Can you work these out from the model? Positions are in its coordinate system, mm. A direction names the side the tool comes from. Round coordinates to 2 decimals unless told otherwise and drop trailing zeros. Order: outer loops, then holes, each group sorted by start corner. A loop starts at its lowest first (then second) coordinate and runs counter-clockwise, first axis right, second up. Notation, with made-up numbers: M -33.75,20 L -20.75,20 A6 cw -20.75,27 Z; hole C -12,60 d1. An arc over 180 degrees is marked long. One line per question, with ' | ' between items.
Autodesk Inventor part; units mm, degrees
ref_plane "YZ Plane" through (0, 0, 0) normal (1, 0, 0) x (0, 1, 0)
ref_plane "XZ Plane" through (0, 0, 0) normal (0, 1, 0) x (-1, 0, 0)
ref_plane "XY Plane" through (0, 0, 0) normal (0, 0, 1) x (1, 0, 0)
sketch "Sketch1" plane through (0, 0, 0) normal (0, 0, 1) x (1, 0, 0)
  line L0 (0, 0) -> (0, -43.18)
  line L1 (0, 0) -> (12.2773, 16)
  line L2 (0, 0) -> (20.1676, 0) construction
  circle A0 centre (12.2773, 16) radius 1.651
  circle A1 centre (0, 0) radius 1.651
  line L3 (10.0328, 17.2474) -> (-2.54, 0.8622)
  line L4 (-2.54, 0.8622) -> (-2.54, -43.18)
  line L5 (14.063, 14.1549) -> (2.54, -0.8622)
  line L6 (2.54, -0.8622) -> (2.54, -43.18)
  line L7 (10.0328, 17.2474) -> (11.9656, 19.7663)
  line L8 (11.9656, 19.7663) -> (15.9959, 16.6738)
  line L9 (15.9959, 16.6738) -> (14.063, 14.1549)
  line L10 (-2.54, -43.18) -> (2.54, -43.18)
  dimension "d0" = 43.18
  dimension "d1" = 20.1676
  dimension "d2" = 52.5
  dimension "d3" = 3.302
  dimension "d4" = 3.302
  dimension "d5" = 2.54
  dimension "d6" = 2.54
  dimension "d7" = 3.175
extrude "Extrusion1" add sketch "Sketch1" along normal blind 5.9182
fillet "Fillet1" radius 3.175 6 edges at (11.9656, 19.7663, 2.9591) (15.9959, 16.6738, 2.9591) (-2.54, 0.8622, 2.9591) (2.54, -0.8622, 2.9591) (2.54, -43.18, 2.9591) (-2.54, -43.18, 2.9591)
sketch "Sketch2" plane through (0, 0, 0) normal (0, 0, -1) x (-1, 0, 0)
  line L0 (-2.54, -40.005) -> (-2.54, -1.94)
  line L1 (-2.54, -11.43) -> (2.54, -11.43)
  line L2 (2.54, -0.2156) -> (2.54, -40.2701)
  arc A0 (-2.54, -40.005) -> (0.635, -43.18) centre (0.635, -40.005) ccw
  circle A1 centre (0, 0) radius 1.651
  circle A2 centre (-12.2773, 16) radius 1.651
  arc A3 (0.635, -43.18) -> (2.54, -40.2701) centre (-0.635, -40.2701) ccw
  line L3 (2.54, -0.2156) -> (2.54, -40.2701)
  arc A4 (2.54, -0.2156) -> (1.8839, 1.7173) centre (-0.635, -0.2156) ccw
  line L4 (-10.0328, 17.2474) -> (1.8839, 1.7173)
  arc A5 (-10.0328, 17.2474) -> (-14.4845, 17.8335) centre (-12.5517, 15.3146) ccw
  arc A6 (-14.4845, 17.8335) -> (-14.2244, 14.3652) centre (-11.7055, 16.298) ccw
  line L5 (-3.1961, -0.0072) -> (-14.2244, 14.3652)
  arc A7 (-2.54, -1.94) -> (-3.1961, -0.0072) centre (-5.715, -1.94) ccw
  line L6 (-2.54, -40.005) -> (-2.54, -1.94)
  arc A8 (-2.54, -40.005) -> (0.635, -43.18) centre (0.635, -40.005) ccw
  point P0 (0.635, -43.18)
  dimension "d11" = 31.75
extrude "Extrusion2" add sketch "Sketch2" along normal blind 8.255 contours L0 L1 L2 A3 A0
fillet "Fillet2" radius 3.175 2 edges at (0, -11.43, 0) (0, -11.43, -8.255)
sketch "Sketch3" plane through (2.54, -40.005, 5.9182) normal (1, 0, 0) x (0, 0, -1)
  circle A0 centre (5.9182, 1.6434) radius 2
  circle A1 centre (5.9182, 25.1399) radius 2
  arc A2 (14.1732, 25.4) -> (10.9982, 28.575) centre (10.9982, 25.4) ccw
  line L0 (9.0932, 28.575) -> (10.9982, 28.575)
  arc A3 (5.9182, 31.75) -> (9.0932, 28.575) centre (9.0932, 31.75) ccw
  line L1 (5.9182, 31.75) -> (5.9182, 38.065)
  line L2 (0, 38.065) -> (5.9182, 38.065)
  line L3 (0, 0) -> (0, 38.065)
  line L4 (0, 0) -> (14.1732, 0)
  line L5 (14.1732, 25.4) -> (14.1732, 0)
  circle A4 centre (10.9982, 12.7) radius 2
  line L6 (5.9182, 1.6434) -> (10.9982, 12.7)
  line L7 (10.9982, 12.7) -> (5.9182, 25.1399)
  line L8 (4.9924, 24.7618) -> (9.9085, 12.7234)
  line L9 (9.9085, 12.7234) -> (5.0095, 2.0609)
  line L10 (6.844, 25.518) -> (12.0879, 12.6766)
  line L11 (12.0879, 12.6766) -> (6.8269, 1.2259)
  point P0 (5.9182, 40.005)
  point P1 (5.6472, 23.1583)
  point P2 (9.4176, 13.9254)
  point P3 (9.3664, 11.5436)
  point P4 (5.7326, 3.6348)
  point P5 (7.55, 2.7998)
  point P6 (11.1838, 10.7086)
  point P7 (11.2692, 14.6816)
  point P8 (7.4988, 23.9144)
  dimension "d15" = 4
  dimension "d16" = 4
  dimension "d17" = 4
  dimension "d18" = 1
  dimension "d19" = 1
extrude "Extrusion3" cut sketch "Sketch3" against normal blind 1 contours A0 L4 | A0 L6 A4 L11 | A0 L4 | A0 L9 A4 L6 | L11 L10 A4 | A4 L6 L7 L10 L11 | A4 L9 L8 L7 L6 | A4 L8 L9 | A4 L7 A1 L10 | L8 A1 L7 A4 | A1
properties part number "Hank - claw"
(1) If we section it at C-C on z = -4.25: Please give me the cut outline in (x, y) (3 decimals), plus the area to 3 significant figures.
Final values:
outline: M -2.54,-40.27 A3.175 ccw -0.635,-43.18 A3.175 ccw 2.54,-40.005 L 2.54,-31.507 L 1.54,-31.507 L 1.54,-22.627 L 2.54,-22.627 L 2.54,-11.43 L -2.54,-11.43 Z | area: 149 mm^2
(2) If we section it at D-D on y = 9: Please give me the cut outline in (x, z), plus the area to 3 significant figures.
Final values:
outline: M 3.7,0 L 10.11,0 L 10.11,5.92 L 3.7,5.92 Z | area: 37.9 mm^2
(3) If we section it at A-A on y = 16: Please give me the cut outline in (x, z), plus the area to 3 significant figures.
Final values:
outline: M 9.08,0 L 10.63,0 L 10.63,5.92 L 9.08,5.92 Z; M 13.93,0 L 14.87,0 L 14.87,5.92 L 13.93,5.92 Z | area: 14.7 mm^2
(4) On a 3-axis mill with a long thin cutter (end or side, diameter ignored), from which of +Z, -Z, +X, -X, +Y, -Y can I reach the whole of each face in a straight line? I mean faces 1 (the cylindrical face through (-2.376, 0.791, 2.918)), 2 (the flat face through (2.54, -21, -1)), 3 (the cylindrical face through (12.103, 18.458, 2.918)), 4 (the flat face through (2.047, -32.36, -1.657)), 5 (the flat face through (0, -11.43, -4)). Say none if no direction works.
Final values:
face 1: +Z, -Z, -X, +Y | face 2: +Z, -Z, +X, -Y | face 3: +Z, -Z, +Y | face 4: +X | face 5: -Z, +X, -X, +Y
(5) If we section it at B-B on x = 0: Please give me the cut outline in (y, z) (3 decimals), plus the area to 3 significant figures.
Final values:
outline: M -43.116,-8.255 L -14.605,-8.255 A3.175 ccw -11.43,-5.08 L -11.43,-3.175 A3.175 cw -8.255,0 L -1.651,0 L -1.651,5.918 L -43.116,5.918 Z; M 1.651,0 L 4.172,0 L 4.172,5.918 L 1.651,5.918 Z | area: 522 mm^2
(6) Thinking about a two-plate mould opening in Z: for faces 6 (the cylindrical face through (2.704, -0.933, 2.918)), 7 (the cylindrical face through (-0.04, -10.52, -0.95)), 8 (the cylindrical face through (2.05, -27.24, -3.08)), 9 (the flat face through (2.05, -21.4, -1.59)), which applies, released by +Z, released by -Z, zero draft, split by the parting line, or undercut?
Final values:
face 6: zero draft | face 7: released by -Z | face 8: undercut | face 9: undercut
(7) Please list where these lines run through material, in increasing order: probe 1 along X at (y, z) = (0, 4.75); probe 2 along Y at (x, z) = (0, 1.75); probe 3 along X at (y, z) = (-24.5, -6.5). Write a range as [from, to].
Final values:
probe 1: [-2.53, -1.65], [1.65, 3.2] | probe 2: [-43.12, -1.65], [1.65, 4.17] | probe 3: [-2.54, 2.54]
(8) Will these pins go through, and if not, where does the flat tip stop? pin 1 Ø5 at (x, z) = (8.5, 2.5) entering from -Y; pin 2 Ø2 at (x, z) = (0, -4.5) entering from +Y; pin 3 Ø4.5 at (y, z) = (-31.5, -4.5) entering from +X.
Final values:
pin 1: y = 3.65 | pin 2: y = -11.43 | pin 3: x = 2.54
